Input: part model. Units: mm. Frame: model coordinates. Coordinates: 2 decimals unless noted, no trailing zeros. Write each loop counter-clockwise with the first axis right and the second up, starting at its lowest first coordinate (ties: lowest second). Pieces come first, ordered by that corner, then holes. Notation, with made-up numbers: M 28,-12.75 L 48,-12.75 A25 cw 48,5.25 Z; hole C -14,42.25 d9. An arc over 180 degrees is marked long. Use CSV: the item, a comma, the result in double quotes.
```python
from build123d import *

# Parameters (mm, degrees)
CYLINDER1267_R               = 2.2
CYLINDER1267_DEPTH           = 15
CYLINDER1267_PLACEMENT_ANGLE = 22.5
CYLINDER1272_R               = 1
CYLINDER1272_DEPTH           = 20
CYLINDER1272_PLACEMENT_ANGLE = 45
CYLINDER1266_R               = 1
CYLINDER1266_DEPTH           = 20
CYLINDER1277_R               = 1
CYLINDER1277_DEPTH           = 20
CYLINDER1277_PLACEMENT_ANGLE = 135
CYLINDER1269_R               = 1
CYLINDER1269_DEPTH           = 20
CYLINDER1275_R               = 1
CYLINDER1275_DEPTH           = 20
CYLINDER1275_PLACEMENT_ANGLE = 225
CYLINDER1274_R               = 1
CYLINDER1274_DEPTH           = 20
CYLINDER1270_R               = 1
CYLINDER1270_DEPTH           = 20
CYLINDER1270_PLACEMENT_ANGLE = 45
CYLINDER1276_R               = 1
CYLINDER1276_DEPTH           = 20
TUBE051_R                    = 32
TUBE051_R_2                  = 24.5
TUBE051_DEPTH                = 1


with BuildPart() as obj1:
    # Cylinder1267 → Cylinder1267 (new body)
    with BuildSketch(Plane.XY):
        Circle(CYLINDER1267_R)
    extrude(amount=CYLINDER1267_DEPTH)


with BuildPart() as obj1_1:
    # Cylinder1267 placement: moved
    add(obj1.part.moved(Location((12.24587, -29.564145, 20))).rotate(Axis((12.24587, -29.564145, 20), (0, 0, 1)), CYLINDER1267_PLACEMENT_ANGLE))


with BuildPart() as obj2:
    # Cylinder1272 → Cylinder1272 (new body)
    with BuildSketch(Plane.XY):
        Circle(CYLINDER1272_R)
    extrude(amount=CYLINDER1272_DEPTH)


with BuildPart() as obj2_1:
    # Cylinder1272 placement: moved
    add(obj2.part.moved(Location((-19.091883, 19.091883, 19))).rotate(Axis((-19.091883, 19.091883, 19), (0, 0, 1)), CYLINDER1272_PLACEMENT_ANGLE))


with BuildPart() as obj3:
    # Cylinder1266 → Cylinder1266 (new body)
    with BuildSketch(Plane(origin=(-27, 0, 19), x_dir=(0, 1, 0), z_dir=(0, 0, 1))):
        Circle(CYLINDER1266_R)
    extrude(amount=CYLINDER1266_DEPTH)


with BuildPart() as obj4:
    # Cylinder1277 → Cylinder1277 (new body)
    with BuildSketch(Plane.XY):
        Circle(CYLINDER1277_R)
    extrude(amount=CYLINDER1277_DEPTH)


with BuildPart() as obj4_1:
    # Cylinder1277 placement: moved
    add(obj4.part.moved(Location((-19.091883, -19.091883, 19))).rotate(Axis((-19.091883, -19.091883, 19), (0, 0, 1)), CYLINDER1277_PLACEMENT_ANGLE))


with BuildPart() as obj5:
    # Cylinder1269 → Cylinder1269 (new body)
    with BuildSketch(Plane(origin=(0, -27, 19), x_dir=(-1, 0, 0), z_dir=(0, 0, 1))):
        Circle(CYLINDER1269_R)
    extrude(amount=CYLINDER1269_DEPTH)


with BuildPart() as obj6:
    # Cylinder1275 → Cylinder1275 (new body)
    with BuildSketch(Plane.XY):
        Circle(CYLINDER1275_R)
    extrude(amount=CYLINDER1275_DEPTH)


with BuildPart() as obj6_1:
    # Cylinder1275 placement: moved
    add(obj6.part.moved(Location((19.091883, -19.091883, 19))).rotate(Axis((19.091883, -19.091883, 19), (0, 0, 1)), CYLINDER1275_PLACEMENT_ANGLE))


with BuildPart() as obj7:
    # Cylinder1274 → Cylinder1274 (new body)
    with BuildSketch(Plane(origin=(27, 0, 19), x_dir=(0, -1, 0), z_dir=(0, 0, 1))):
        Circle(CYLINDER1274_R)
    extrude(amount=CYLINDER1274_DEPTH)


with BuildPart() as obj8:
    # Cylinder1270 → Cylinder1270 (new body)
    with BuildSketch(Plane.XY):
        Circle(CYLINDER1270_R)
    extrude(amount=CYLINDER1270_DEPTH)


with BuildPart() as obj8_1:
    # Cylinder1270 placement: moved
    add(obj8.part.moved(Location((19.091883, 19.091883, 19))).rotate(Axis((19.091883, 19.091883, 19), (0, 0, -1)), CYLINDER1270_PLACEMENT_ANGLE))


with BuildPart() as compound677:
    # Cylinder1276 → Cylinder1276 (new body)
    with BuildSketch(Plane(origin=(0, 27, 19), x_dir=(1, 0, 0), z_dir=(0, 0, 1))):
        Circle(CYLINDER1276_R)
    extrude(amount=CYLINDER1276_DEPTH)

    # Compound677: union obj2, obj3, obj4, obj5, obj6, obj7, obj8
    add(obj2_1.part)
    add(obj3.part)
    add(obj4_1.part)
    add(obj5.part)
    add(obj6_1.part)
    add(obj7.part)
    add(obj8_1.part)


with BuildPart() as cut479:
    # Tube051 → Tube051 (new body)
    with BuildSketch(Plane.XY.offset(25)):
        Circle(TUBE051_R)
        Circle(TUBE051_R_2, mode=Mode.SUBTRACT)
    extrude(amount=TUBE051_DEPTH)

    # Cut476: cut Compound677
    add(compound677.part, mode=Mode.SUBTRACT)

    # Cut479: cut obj1
    add(obj1_1.part, mode=Mode.SUBTRACT)


solid = cut479.part
```
1. Contact query for a flat-ended pin moving along its axis: pin 1 Ø2.5 at (x, y) = (19.09, 19.09) entering from -Z. Output: stop coordinate, or through.
Resolved:
pin 1,"stops at z = 25"
2. Section D-D (z = 25.8). State how many separate pieces and enclosed holes the cut face has, then the cut area to 3 significant figures.
Resolved:
separate pieces,"1"
enclosed holes,"9"
area,"1,300 mm^2"
3. Section C-C (y = 27). Return loops of the section in (x, z).
Resolved:
outline,"M -17.18,25 L -1,25 L -1,26 L -17.18,26 Z; M 1,25 L 17.18,25 L 17.18,26 L 1,26 Z"
4. Section A-A (y = 0). Return loops of the section in (x, z).
Resolved:
outline,"M -32,25 L -28,25 L -28,26 L -32,26 Z; M -26,25 L -24.5,25 L -24.5,26 L -26,26 Z; M 24.5,25 L 26,25 L 26,26 L 24.5,26 Z; M 28,25 L 32,25 L 32,26 L 28,26 Z"
5. Material intervals for line 1 (Y direction, x = 0, z = 25.65); line 2 (X direction, y = -11, z = 25.9); line 3 (Y direction, x = 5.5, z = 25.4), sorted ascending. Write a range as [from, to].
Resolved:
line 1,"y = [-32, -28], [-26, -24.5], [24.5, 26], [28, 32]"
line 2,"x = [-30.05, -21.89], [21.89, 30.05]"
line 3,"y = [-31.52, -23.87], [23.87, 31.52]"
6. Mould query, pull axis X, two halves, no side actions, for faces 1 (the cylindrical face through (-10.963, 30.063, 25.493)), 2 (the cylindrical face through (0.13, -27.99, 25.49)), 3 (the flat face through (24, 7, 26)). Classes: pulls with the +X half, pulls with the -X half, needs draft (parallel to the pull), parting line crosses it, or undercut.
Resolved:
face 1,"parting line crosses it"
face 2,"undercut"
face 3,"needs draft"
